```python
from build123d import *

# Parameters (mm, degrees)
SKETCH1_W                    = 92.075
SKETCH1_H                    = 15.875
BOSS_EXTRUDE1_DEPTH          = 15.875
CUT_EXTRUDE1_REACH           = 53.22
SKETCH2_W                    = 47.625
SKETCH2_H                    = 15.875
F_10_0_1935_DIAMETER_HOLE1_D = 5.1054
CUT_EXTRUDE2_REACH           = 51.34
SKETCH5_W                    = 47.625
SKETCH5_H                    = 8.255
CUT_EXTRUDE3_REACH           = 51.34
SKETCH6_W                    = 47.625
SKETCH6_H                    = 3.81
SKETCH7_W                    = 38.1
SKETCH7_H                    = 9.525
CUT_EXTRUDE4_DEPTH           = 57.484668827
SKETCH8_W                    = 6.35
SKETCH8_H                    = 3.81
CUT_EXTRUDE5_DEPTH           = 57.484668827
F_10_32_TAPPED_HOLE1_D       = 4.0386
SKETCH11_W                   = 24.765
SKETCH11_H                   = 15.875
BOSS_EXTRUDE2_DEPTH          = 3.81
SKETCH12_W                   = 6.35
SKETCH12_H                   = 15.875
BOSS_EXTRUDE3_DEPTH          = 3.81


with BuildPart() as part:
    # Sketch1 → Boss-Extrude1 (new, symmetric)
    with BuildSketch(Plane(origin=(0, 0, 0), x_dir=(1, 0, 0), z_dir=(0, 1, 0))):
        Rectangle(SKETCH1_W, SKETCH1_H)
    extrude(amount=BOSS_EXTRUDE1_DEPTH, both=True)

    # Sketch2 → Cut-Extrude1 (cut, up to next)
    with BuildSketch(Plane.XY.offset(7.9375), mode=Mode.PRIVATE) as cut_extrude1_sk1:
        with Locations((22.225, 7.9375)):
            Rectangle(SKETCH2_W, SKETCH2_H)
    cut_extrude1_tool1 = extrude(cut_extrude1_sk1.sketch, amount=-CUT_EXTRUDE1_REACH, mode=Mode.PRIVATE) & part.part
    add(cut_extrude1_tool1.solids().sort_by_distance((22.225, 7.9375, 7.9375))[0], mode=Mode.SUBTRACT)

    # #10 (0.1935) Diameter Hole1 (through all)
    with Locations(Plane.XY.offset(7.9375)):
        with Locations((-33.3375, 9.525), (-20.6375, 9.525)):
            Hole(F_10_0_1935_DIAMETER_HOLE1_D / 2)

    # Sketch5 → Cut-Extrude2 (cut, up to next)
    with BuildSketch(Plane(origin=(0, 0, 0), x_dir=(1, 0, 0), z_dir=(0, 1, 0)), mode=Mode.PRIVATE) as cut_extrude2_sk1:
        with Locations((22.225, 3.81)):
            Rectangle(SKETCH5_W, SKETCH5_H)
    cut_extrude2_tool1 = extrude(cut_extrude2_sk1.sketch, amount=-CUT_EXTRUDE2_REACH, mode=Mode.PRIVATE) & part.part
    add(cut_extrude2_tool1.solids().sort_by_distance((22.225, 0, -3.81))[0], mode=Mode.SUBTRACT)

    # Sketch6 → Cut-Extrude3 (cut, up to next)
    with BuildSketch(Plane(origin=(0, 0, 0), x_dir=(1, 0, 0), z_dir=(0, 1, 0)), mode=Mode.PRIVATE) as cut_extrude3_sk1:
        with Locations((22.225, -6.0325)):
            Rectangle(SKETCH6_W, SKETCH6_H)
    cut_extrude3_tool1 = extrude(cut_extrude3_sk1.sketch, amount=-CUT_EXTRUDE3_REACH, mode=Mode.PRIVATE) & part.part
    add(cut_extrude3_tool1.solids().sort_by_distance((22.225, 0, 6.0325))[0], mode=Mode.SUBTRACT)

    # Sketch7 → Cut-Extrude4 (cut, through all)
    with BuildSketch(Plane(origin=(0, 15.875, 0), x_dir=(1, 0, 0), z_dir=(0, 1, 0))):
        with Locations((-26.9875, -3.175)):
            Rectangle(SKETCH7_W, SKETCH7_H)
    extrude(amount=-CUT_EXTRUDE4_DEPTH, mode=Mode.SUBTRACT)

    # Sketch8 → Cut-Extrude5 (cut, through all)
    with BuildSketch(Plane(origin=(0, 15.875, 0), x_dir=(1, 0, 0), z_dir=(0, 1, 0))):
        with Locations((-4.7625, -6.0325)):
            Rectangle(SKETCH8_W, SKETCH8_H)
    extrude(amount=-CUT_EXTRUDE5_DEPTH, mode=Mode.SUBTRACT)

    # #10-32 Tapped Hole1 (through all)
    with Locations(Plane.XY.offset(4.1275)):
        with Locations((39.6875, -7.9375), (26.9875, -7.9375)):
            Hole(F_10_32_TAPPED_HOLE1_D / 2)

    # Sketch11 → Boss-Extrude2 (add)
    with BuildSketch(Plane.XY.offset(4.1275)):
        with Locations((4.445, -7.9375)):
            Rectangle(SKETCH11_W, SKETCH11_H)
    extrude(amount=BOSS_EXTRUDE2_DEPTH)

    # Sketch12 → Boss-Extrude3 (add)
    with BuildSketch(Plane.XY.offset(4.1275)):
        with Locations((-4.7625, 7.9375)):
            Rectangle(SKETCH12_W, SKETCH12_H)
    extrude(amount=BOSS_EXTRUDE3_DEPTH)


solid = part.part
```
Part model, mm, in its own coordinate system. A direction names the side the tool comes from. Round coordinates to 2 decimals unless told otherwise and drop trailing zeros. Order: outer loops, then holes, each group sorted by start corner. A loop starts at its lowest first (then second) coordinate and runs counter-clockwise, first axis right, second up. Notation, with made-up numbers: M 4.5,20.5 L 53.5,20.5 A8 cw 53.5,27.5 Z; hole C 13,-14.5 d5. An arc over 180 degrees is marked long. Answer in a Markdown table with one row per item. Add a question column.
Q1. Pin check, flat tips, straight feed: pin 1 (1.5 mm diameter, centred on y = 5.5, z = 5, fed in from -X); pin 2 (6.5 mm diameter, centred on x = 26.99, y = -7.94, fed in from -Z); pin 3 (17.5 mm diameter, centred on x = 24.5, y = -11, fed in from +Z); pin 4 (2 mm diameter, centred on y = -12, z = -4.5, fed in from +X). Stop position of each tip, or through.
Q2. Cut at C-C on y = 11. Give the cut face in (x, z).
Q3. Mould opens along Y. For faces 1 (the face through (-1.588, 3, -2)), 2 (the face through (17, 0, 3)), 3 (the face through (-22.996, 8.547, -4.807)) say: +Y half, -Y half, draft (parallel to the pull), parting line (faces both ways), or undercut.
Q4. 3-axis set-ups, long thin cutter, end or side, ignore diameter. For faces 4 (the face through (16.828, -8, 6)), 5 (the face through (22, -8, 0.318)), 6 (the face through (-46.038, 0, -5)), 7 (the face through (-27, 0, -1.588)): which of +Z, -Z, +X, -X, +Y, -Y reach the whole face in a straight line?
Q5. Cut at D-D on x = 40.5. Give the cut face in (y, z) (1 decimal), and give its area (3 significant figures).
Q6. Cut at A-A on z = 1.75. Give the cut face in (x, y) (1 decimal).
Q7. Cut at B-B on y = -5. Give the cut face in (x, z).
Q8. Wall check: L1, parallel to X at y = -11.5, z = 4.5; L2, parallel to Z at x = -29, y = -14; L3, parallel to X at y = 4, z = -6.5. Give the ranges that are in metal, low to high. Write a range as from..to.
Established:
| question | item | result |
|---|---|---|
| 1 | pin 1 | stops at x = -7.94 |
| 1 | pin 2 | stops at z = 0.32 |
| 1 | pin 3 | stops at z = 7.94 |
| 1 | pin 4 | stops at x = -1.59 |
| 2 | outline | M -46.04,-7.94 L -35.42,-7.94 L -35.42,-1.59 L -46.04,-1.59 Z; M -31.25,-7.94 L -22.72,-7.94 L -22.72,-1.59 L -31.25,-1.59 Z; M -18.55,-7.94 L -1.59,-7.94 L -1.59,7.94 L -7.94,7.94 L -7.94,-1.59 L -18.55,-1.59 Z |
| 3 | face 1 | draft |
| 3 | face 2 | +Y half |
| 3 | face 3 | undercut |
| 4 | face 4 | +Z, +X, +Y, -Y |
| 4 | face 5 | -Z, +X, +Y, -Y |
| 4 | face 6 | +Z, -Z, -X, +Y, -Y |
| 4 | face 7 | +Z, -X, +Y, -Y |
| 5 | outline | M -15.9,0.3 L -9.8,0.3 L -9.8,4.1 L -15.9,4.1 Z; M -6.1,0.3 L 0,0.3 L 0,4.1 L -6.1,4.1 Z |
| 5 | area | 46.4 mm2 |
| 6 | outline | M -7.9,-15.9 L 46,-15.9 L 46,0 L -1.6,0 L -1.6,15.9 L -7.9,15.9 Z; hole C 27,-7.9 d4; hole C 39.7,-7.9 d4 |
| 7 | outline | M -46.04,-7.94 L -1.59,-7.94 L -1.59,0.32 L 46.04,0.32 L 46.04,4.13 L 16.83,4.13 L 16.83,7.94 L -7.94,7.94 L -7.94,-1.59 L -46.04,-1.59 Z |
| 8 | L1 | x = -7.94..16.83 |
| 8 | L2 | z = -7.94..-1.59 |
| 8 | L3 | x = -46.04..-1.59 |
